Read the model definition and answer for the solid it produces. Units are mm, in the model's axes. A direction names the side the tool comes from. Coordinates: 2 decimals unless noted, no trailing zeros. Order: outer loops, then holes, each group sorted by start corner. A loop starts at its lowest first (then second) coordinate and runs counter-clockwise, first axis right, second up. Notation, with made-up numbers: (65, -13.5) -> (100, -13.5) arc R16 cw to (100, -4.5) -> close; hole circle Ø11 at (46, 75.25). An arc over 180 degrees is marked (long way). Answer in a Markdown table with one row per item.
from build123d import *

# Parameters (mm, degrees)
SKETCH_1_R      = 1.7
EXTRUDE_1_DEPTH = 5


with BuildPart() as part:
    # 草图1 → 凸台-拉伸1 (new body)
    with BuildSketch(Plane(origin=(0, 0, 0), x_dir=(1, 0, 0), z_dir=(0, 1, 0))):
        Polygon((2550.050393087, 1533.227125386), (2557.121460899, 1540.298193198), (2574.979325275, 1540.298193198), (2582.050393087, 1533.227125386), (2582.050393087, 1413.227125386), (2574.979325275, 1406.156057575), (2557.121460899, 1406.156057575), (2550.050393087, 1413.227125386), align=None)
        with Locations(Location((2571.050393087, 1483.227125386, 0), (0, 0, 270))):
            Circle(SKETCH_1_R, mode=Mode.SUBTRACT)
        with Locations(Location((2561.050393087, 1483.227125386, 0), (0, 0, 270))):
            Circle(SKETCH_1_R, mode=Mode.SUBTRACT)
        with Locations(Location((2561.050393087, 1463.227125386, 0), (0, 0, 270))):
            Circle(SKETCH_1_R, mode=Mode.SUBTRACT)
        with Locations(Location((2571.050393087, 1463.227125386, 0), (0, 0, 270))):
            Circle(SKETCH_1_R, mode=Mode.SUBTRACT)
        with BuildLine():
            Line((2576.250393087, 1487.527125386), (2555.850393087, 1487.527125386))
            Line((2555.850393087, 1487.527125386), (2555.850393087, 1527.927125386))
            Line((2555.850393087, 1527.927125386), (2559.850393087, 1527.927125386))
            Line((2559.850393087, 1527.927125386), (2561.368882267, 1530.557225796))
            ThreePointArc((2561.368882267, 1530.557225796), (2559.578149901, 1533.077125386), (2562.655813144, 1532.786255462))
            Line((2562.655813144, 1532.786255462), (2563.850393087, 1534.855328617))
            Line((2563.850393087, 1534.855328617), (2568.250393087, 1534.855328617))
            Line((2568.250393087, 1534.855328617), (2569.44497303, 1532.786255462))
            ThreePointArc((2569.44497303, 1532.786255462), (2572.522636274, 1533.077125386), (2570.731903908, 1530.557225796))
            Line((2570.731903908, 1530.557225796), (2572.250393087, 1527.927125386))
            Line((2572.250393087, 1527.927125386), (2576.250393087, 1527.927125386))
            Line((2576.250393087, 1527.927125386), (2576.250393087, 1487.527125386))
        make_face(mode=Mode.SUBTRACT)
        with BuildLine():
            Line((2555.850393087, 1458.927125386), (2576.250393087, 1458.927125386))
            Line((2576.250393087, 1458.927125386), (2576.250393087, 1418.527125386))
            Line((2576.250393087, 1418.527125386), (2572.250393087, 1418.527125386))
            Line((2572.250393087, 1418.527125386), (2570.731903908, 1415.897024977))
            ThreePointArc((2570.731903908, 1415.897024977), (2572.522636274, 1413.377125386), (2569.44497303, 1413.667995311))
            Line((2569.44497303, 1413.667995311), (2568.250393087, 1411.598922156))
            Line((2568.250393087, 1411.598922156), (2563.850393087, 1411.598922156))
            Line((2563.850393087, 1411.598922156), (2562.655813144, 1413.667995311))
            ThreePointArc((2562.655813144, 1413.667995311), (2559.578149901, 1413.377125386), (2561.368882267, 1415.897024977))
            Line((2561.368882267, 1415.897024977), (2559.850393087, 1418.527125386))
            Line((2559.850393087, 1418.527125386), (2555.850393087, 1418.527125386))
            Line((2555.850393087, 1418.527125386), (2555.850393087, 1458.927125386))
        make_face(mode=Mode.SUBTRACT)
    extrude(amount=EXTRUDE_1_DEPTH)


solid = part.part
Q1. The part is cut by section A-A (z = -1489.5). Write down the section's boundary in (x, y), then the cut area to 3 significant figures.
Outcome:
| item | result |
|---|---|
| outline | (2550.05, 0) -> (2555.85, 0) -> (2555.85, 5) -> (2550.05, 5) -> close; (2576.25, 0) -> (2582.05, 0) -> (2582.05, 5) -> (2576.25, 5) -> close |
| area | 58.0 mm² |
Q2. Given pin 1 (4.5 mm diameter, centred on x = 2561.05, z = -1463.23, fed in from +Y), flat-ended and moving along its own axis, determine where the tip first touches the part or whether it passes through.
Outcome:
| item | result |
|---|---|
| pin 1 | y = 5 |
Q3. The part is cut by section C-C (x = 2580). Write down the section's boundary in (y, z), then the cut area to 3 significant figures.
Outcome:
| item | result |
|---|---|
| outline | (0, -1535.28) -> (5, -1535.28) -> (5, -1411.18) -> (0, -1411.18) -> close |
| area | 621 mm² |
Q4. For faces 4 (the face through (2578.47, 2.46, -1536.81)), 5 (the face through (2566, 2, -1411.599)), determine the directions among +Z, -Z, +X, -X, +Y, -Y from which every point of the face is accessible in a straight line to the end or side of a thin tool.
Outcome:
| item | result |
|---|---|
| face 4 | -Z, +X, +Y, -Y |
| face 5 | +Y, -Y |
Q5. The part is cut by section B-B (y = 1). Give the number of separate pieces and of enclosed holes in the cut face, then the cut area to 3 significant figures.
Outcome:
| item | result |
|---|---|
| separate pieces | 1 |
| enclosed holes | 6 |
| area | 2,360 mm² |
Q6. Consider line 1 (Z direction, x = 2575, y = 0.4); line 2 (Z direction, x = 2566, y = 1.4); line 3 (X direction, y = 1.45, z = -1449). Determine where each line is inside the solid, lowest interval first.
Outcome:
| item | result |
|---|---|
| line 1 | -1540.28 to -1527.93, -1487.53 to -1458.93, -1418.53 to -1406.18 |
| line 2 | -1540.3 to -1534.86, -1487.53 to -1458.93, -1411.6 to -1406.16 |
| line 3 | 2550.05 to 2555.85, 2576.25 to 2582.05 |
Q7. For a pull along Z with two mould halves and no side action, classify faces 1 (the face through (2566, 2, -1406.156)), 2 (the face through (2553.536, 2.465, -1536.713)), 3 (the face through (2566, 2, -1487.527)) as pulls with the +Z half, pulls with the -Z half, needs draft (parallel to the pull), parting line crosses it, or undercut.
Outcome:
| item | result |
|---|---|
| face 1 | pulls with the +Z half |
| face 2 | pulls with the -Z half |
| face 3 | undercut |
